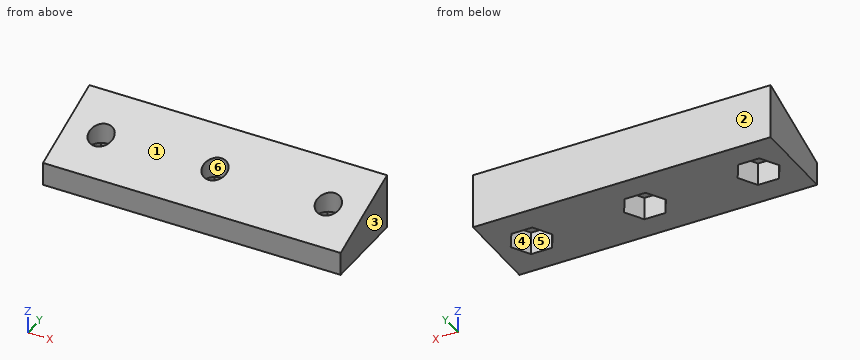
Solid Edge part; units mm, degrees
sketch "Sketch1" plane through (0, 0, -17) normal (0, 0, -1) x (-1, 0, 0)
  circle A0 centre (30.5803, -5.7499) radius 2.6398
  line L0 (38.3399, -15.0506) -> (-27.2379, -15.0506)
  line L1 (-27.2379, -15.0506) -> (-27.2379, 3.7685)
  line L2 (-27.2379, 3.7685) -> (38.3399, 3.7685)
  line L3 (38.3399, 3.7685) -> (38.3399, -15.0506)
  circle A1 centre (5.551, -5.6411) radius 2.6333
  circle A2 centre (-19.4978, -5.7928) radius 2.6563
extrude "Protrusion1" add sketch "Sketch1" against normal blind 13
sketch "Sketch2" plane through (-38.3399, -5.6411, -10.5) normal (-1, 0, 0) x (0, 1, 0)
  line L0 (-9.4095, 1.3904) -> (9.4095, -5.6409)
  line L1 (9.4095, -6.5) -> (9.4095, -5.6409)
  line L2 (9.4095, -6.5) -> (-9.4095, -6.5)
  line L3 (-9.4095, -6.5) -> (-9.4095, 1.3904)
extrude "ExtrudedCutout_1" cut sketch "Sketch2" against normal blind 81
sketch "Sketch3" plane through (-5.551, -5.6411, -17) normal (0, 0, -1) x (0, 1, 0)
  circle A0 centre (0, 0) radius 2.6333
  line L0 (0, -4.6188) -> (4, -2.3094)
  line L1 (4, -2.3094) -> (4, 2.3094)
  line L2 (4, 2.3094) -> (0, 4.6188)
  line L3 (0, 4.6188) -> (-4, 2.3094)
  line L4 (-4, 2.3094) -> (-4, -2.3094)
  line L5 (-4, -2.3094) -> (0, -4.6188)
  circle A1 centre (-0.1517, 25.0488) radius 2.6563
  line L6 (-0.1517, 20.43) -> (3.8483, 22.7394)
  line L7 (3.8483, 22.7394) -> (3.8483, 27.3582)
  line L8 (3.8483, 27.3582) -> (-0.1517, 29.6676)
  line L9 (-0.1517, 29.6676) -> (-4.1517, 27.3582)
  line L10 (-4.1517, 27.3582) -> (-4.1517, 22.7394)
  line L11 (-4.1517, 22.7394) -> (-0.1517, 20.43)
  circle A2 centre (-0.1089, -25.0293) radius 2.6398
  line L12 (-4, -27.3387) -> (0, -29.6481)
  line L13 (0, -29.6481) -> (4, -27.3387)
  line L14 (4, -27.3387) -> (4, -22.7199)
  line L15 (4, -22.7199) -> (0, -20.4105)
  line L16 (0, -20.4105) -> (-4, -22.7199)
  line L17 (-4, -22.7199) -> (-4, -27.3387)
extrude "ExtrudedCutout_2" cut sketch "Sketch3" against normal blind 5
The listing builds one solid part. Answer for the finished solid, in the listing's coordinates (mm). Face numbers are marked on the shaded views. A direction names the side the tool comes from. Coordinates: 2 decimals unless noted, no trailing zeros. Write each loop counter-clockwise with the first axis right and the second up, starting at its lowest first coordinate (ties: lowest second). Pieces come first, ordered by that corner, then holes. Notation, with made-up numbers: M -19.75,73.25 L -0.75,73.25 A31 ccw -0.75,97.25 Z; hole C 31.25,-10 d5. An arc over 180 degrees is marked long. Use a Markdown table: item, result. Add a question column.
1. Section D-D (x = 11.5) is taken. Give the vertices of the cut face in (y, z), plus the area to 3 significant figures.
2. Which of the six approach directions +Z, -Z, +X, -X, +Y, -Y give full straight-line access (tool end or side, diameter ignored) to the marked faces 5 and 6?
3. Section C-C (x = 19.5) is taken. Give the vertices of the cut face in (y, z), plus the area to 3 significant figures.
4. Straight lines are drawn through the part: line 1 along Y through (x, z) = (-7.5, -12.75); line 2 along X through (y, z) = (-6.5, -9.25); line 3 along X through (y, z) = (-3.5, -14.5). For each, find the intervals that lie inside material, in ascending order. Write a range as [from, to].
5. Given P1, Ø6, axis at x = 19.5, y = -5.79, coming from the -Z side; P2, Ø6, axis at x = -5.55, y = -5.64, coming from the +Z side; P3, Ø1.5, axis at x = 0, y = -4.5, coming from the +Z side; P4, Ø5, axis at y = -12, z = -7.5, coming from the -X side, each flat-ended and moving along its own axis, determine where each tip first touches the part or whether it passes through.
6. For a pull along Y with two mould halves and no side action, classify the marked faces 1, 2, 3 and 4 as +Y half, -Y half, draft (parallel to the pull), parting line (faces both ways), or undercut.
7. Section A-A (z = -15.25) is taken. Give the vertices of the cut face in (x, y), plus the area to 3 significant figures.
8. Section B-B (y = -4) is taken. Give the vertices of the cut face in (x, z).
Data:
| question | item | result |
|---|---|---|
| 1 | outline | M -15.05,-17 L 3.77,-17 L 3.77,-4.86 L -15.05,-11.89 Z |
| 1 | area | 162 mm2 |
| 2 | face 5 | -Z |
| 2 | face 6 | +Z, -Z |
| 3 | outline | M -15.05,-17 L -9.79,-17 L -9.79,-12 L -8.45,-12 L -8.45,-9.42 L -15.05,-11.89 Z; M -3.14,-12 L -1.79,-12 L -1.79,-17 L 3.77,-17 L 3.77,-4.86 L -3.14,-7.44 Z |
| 3 | area | 103 mm2 |
| 4 | line 1 | y = [-15.05, -9.64], [-1.64, 3.77] |
| 4 | line 2 | x = [-38.34, -33.11], [-28.05, -8.04], [-3.06, 16.94], [22.06, 27.24] |
| 4 | line 3 | x = [-38.34, -33.96], [-27.2, -8.93], [-2.17, 16.2], [22.79, 27.24] |
| 5 | P1 | stops at z = -12 |
| 5 | P2 | stops at z = -7.25 |
| 5 | P3 | stops at z = -7.67 |
| 5 | P4 | passes through |
| 6 | face 1 | -Y half |
| 6 | face 2 | +Y half |
| 6 | face 3 | draft |
| 6 | face 4 | undercut |
| 7 | outline | M -38.34,-15.05 L 27.24,-15.05 L 27.24,3.77 L -38.34,3.77 Z; hole M -35.2,-5.64 L -32.89,-9.64 L -28.27,-9.64 L -25.96,-5.64 L -28.27,-1.64 L -32.89,-1.64 Z; hole M -10.17,-5.64 L -7.86,-9.64 L -3.24,-9.64 L -0.93,-5.64 L -3.24,-1.64 L -7.86,-1.64 Z; hole M 14.88,-5.79 L 17.19,-9.79 L 21.81,-9.79 L 24.12,-5.79 L 21.81,-1.79 L 17.19,-1.79 Z |
| 7 | area | 1,070 mm2 |
| 8 | outline | M -38.34,-17 L -34.25,-17 L -34.25,-12 L -32.56,-12 L -32.56,-7.76 L -38.34,-7.76 Z; M -28.6,-12 L -26.91,-12 L -26.91,-17 L -9.22,-17 L -9.22,-12 L -7.61,-12 L -7.61,-7.76 L -28.6,-7.76 Z; M -3.49,-12 L -1.88,-12 L -1.88,-17 L 15.91,-17 L 15.91,-12 L 17.54,-12 L 17.54,-7.76 L -3.49,-7.76 Z; M 21.46,-12 L 23.08,-12 L 23.08,-17 L 27.24,-17 L 27.24,-7.76 L 21.46,-7.76 Z |
